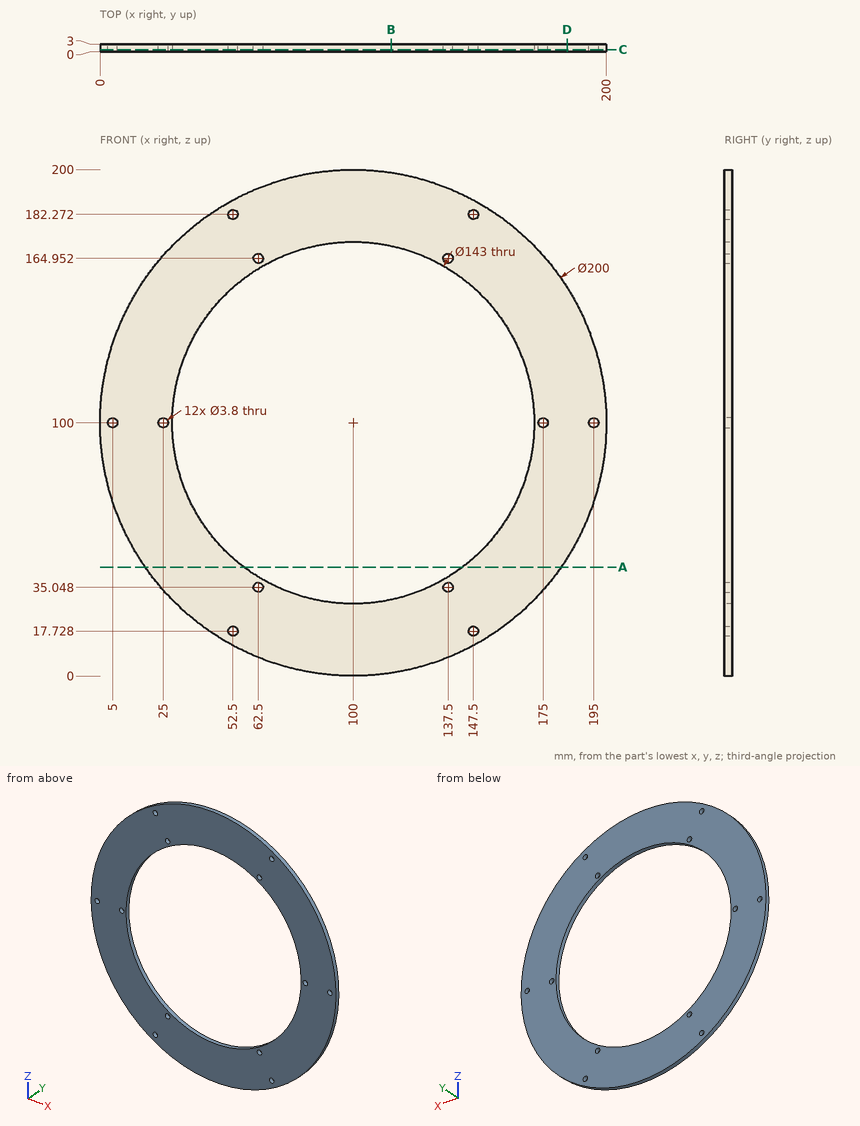
Input: dimensioned drawing with shaded views. Units: mm. Origin: part minimum x, y, z. Round coordinates to 2 decimals unless told otherwise and drop trailing zeros. Order: outer loops, then holes, each group sorted by start corner. A loop starts at its lowest first (then second) coordinate and runs counter-clockwise, first axis right, second up. Notation, with made-up numbers: (-20.75, 79) -> (4.25, 79) arc R31 ccw to (4.25, 113) -> close; hole circle Ø10 at (30.5, 80.5). An arc over 180 degrees is marked (long way). Put each result on its own line as item: value. Start each with the question number.
Q1. Section C-C on y = 0.8. Give the number of separate pieces and of enclosed holes in the cut face, and give its area (3 significant figures).
Q2. First-contact query: pin 1 (1 mm diameter, centred on y = 1.5, z = 45, fed in from +X); pin 2 (1 mm diameter, centred on y = 2.5, z = 73, fed in from +X) (1 decimal). Flat tips, straight axial feed; report the tip coordinate or a pass-through.
Q3. Line query: probe 1 along X at (y, z) = (2, 100); probe 2 along X at (y, z) = (1.2, 107) (1 decimal); probe 3 along Z at (x, y) = (158.5, 1.85) (1 decimal). Output: solid intervals per line, ascending.
Q4. Section D-D on x = 184.5. Return the cut outline in (y, z).
Q5. Section A-A on z = 43. Return the cut outline in (x, y) (1 decimal), and give its area (3 significant figures).
Q6. Section B-B on x = 115. Return the cut outline in (y, z).
Ans:
1. separate pieces: 1
1. enclosed holes: 13
1. area: 15,200 mm2
2. pin 1: stops at x = 183.84
2. pin 2: stops at x = 196.4
3. probe 1: x = 0 to 3.1, 6.9 to 23.1, 26.9 to 28.5, 171.5 to 173.1, 176.9 to 193.1, 196.9 to 200
3. probe 2: x = 0.2 to 28.8, 171.2 to 199.8
3. probe 3: z = 18.9 to 58.9, 141.1 to 181.1
4. outline: (0, 46.52) -> (3, 46.52) -> (3, 153.48) -> (0, 153.48) -> close
5. outline: (17.8, 0) -> (56.8, 0) -> (56.8, 3) -> (17.8, 3) -> close; (143.2, 0) -> (182.2, 0) -> (182.2, 3) -> (143.2, 3) -> close
5. area: 234 mm2
6. outline: (0, 1.13) -> (3, 1.13) -> (3, 30.09) -> (0, 30.09) -> close; (0, 169.91) -> (3, 169.91) -> (3, 198.87) -> (0, 198.87) -> close
